Part print with two shaded views. Sizes in mm from the minimum x, y, z corner. Round coordinates to 2 decimals unless told otherwise and drop trailing zeros. Loops run counter-clockwise (first coordinate to the right, second up) from the corner with the lowest first, then second, coordinate; pieces in that order, holes last.
(1) Cut at B-B on x = 16.5. List the corners of the cut face in (y, z).
(2) Cut at A-A on z = 5. List the corners of the cut face in (x, y).
(3) Flat gauge pins, fed straight in: pin 1 (5 mm diameter, centred on y = 15, z = 12, fed in from -X); pin 2 (10 mm diameter, centred on x = 4, y = 7.5, fed in from -Z); pin 3 (6 mm diameter, centred on x = 2.5, z = 5, fed in from +Y); pin 4 (10 mm diameter, centred on x = 10, y = 5.5, fed in from -Z). Where does each tip first touch, or does it go through?
(4) Probe probe 1 along Y at (x, z) = (8.5, 7.75); probe 2 along Y at (x, z) = (5.5, 10.25); probe 3 along Z at (x, y) = (1.5, 9.75). List the from-to ranges inside material, lowest first.
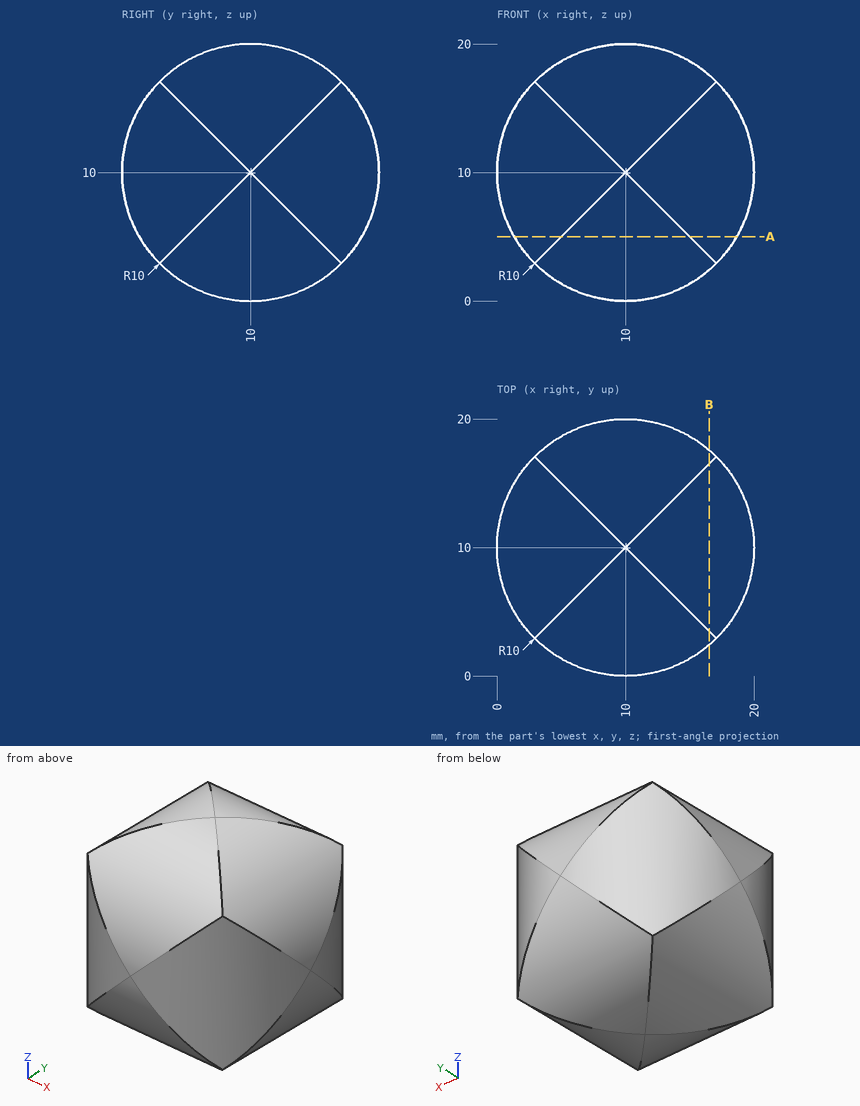
Final values:
1. outline: (2.4, 3.5) arc R10 ccw to (3.5, 2.4) - (16.5, 2.4) arc R10 ccw to (17.6, 3.5) - (17.6, 16.5) arc R10 ccw to (16.5, 17.6) - (3.5, 17.6) arc R10 ccw to (2.4, 16.5) - close
2. outline: (1.34, 5) arc R10 ccw to (5, 1.34) - (15, 1.34) arc R10 ccw to (18.66, 5) - (18.66, 15) arc R10 ccw to (15, 18.66) - (5, 18.66) arc R10 ccw to (1.34, 15) - close
3. pin 1: stops at x = 0.32
3. pin 2: stops at z = 0.07
3. pin 3: stops at y = 18.91
3. pin 4: stops at z = 0
4. probe 1: y = 0.26 to 19.74
4. probe 2: y = 1.07 to 18.93
4. probe 3: z = 4.73 to 15.27
